from build123d import *

# Parameters (mm, degrees)
BOSS_EXTRUDE1_DEPTH = 5
SKETCH2_W           = 1.6
SKETCH2_H           = 1.6
CUT_EXTRUDE1_DEPTH  = 0.3
FILLET1_R           = 0.5


with BuildPart() as part:
    # Sketch1 → Boss-Extrude1 (new body)
    with BuildSketch(Plane(origin=(0, 0, 0), x_dir=(0, 0, -1), z_dir=(1, 0, 0))):
        with BuildLine():
            Line((-5.181029882, 3.015192247), (-4, 2.806944814))
            Line((-4, 2.806944814), (0.163235541, 2.072854061))
            ThreePointArc((0.163235541, 2.072854061), (0.459433673, 1.901843989), (0.576411452, 1.580450184))
            Line((0.576411452, 1.580450184), (0.576411452, 1.5))
            ThreePointArc((0.576411452, 1.5), (0.429964842, 1.146446609), (0.076411452, 1))
            Line((0.076411452, 1), (-6.25, 1))
            Line((-6.25, 1), (-6.25, 0))
            Line((-6.25, 0), (-4.8, 0))
            Line((-4.8, 0), (-4.8, -0.3))
            Line((-4.8, -0.3), (-3.2, -0.3))
            Line((-3.2, -0.3), (-3.2, 0))
            Line((-3.2, 0), (-1, 0))
            Line((-1, 0), (-1, -0.5))
            Line((-1, -0.5), (0, -0.5))
            Line((0, -0.5), (0, 0))
            ThreePointArc((0, 0), (1.536997065, 1.222015685), (0.692851848, 2.994895028))
            Line((0.692851848, 2.994895028), (-5.007381704, 4))
            Line((-5.007381704, 4), (-5.181029882, 3.015192247))
        make_face()
    extrude(amount=BOSS_EXTRUDE1_DEPTH)

    # Sketch2 → Cut-Extrude1 (cut)
    with BuildSketch(Plane.XZ.offset(0.3)):
        with Locations((2.5, 4)):
            Rectangle(SKETCH2_W, SKETCH2_H)
    extrude(amount=-CUT_EXTRUDE1_DEPTH, mode=Mode.SUBTRACT)

    # Fillet1
    fillet1_edges = [part.edges().sort_by_distance(p)[0] for p in [
        (0, 0.5, 6.25),
        (0, 3.507596123, 5.094205793),
        (5, 3.507596123, 5.094205793),
        (5, 0.5, 6.25),
    ]]
    fillet(fillet1_edges, radius=FILLET1_R)


solid = part.part
Part model, mm, in its own coordinate system. A direction names the side the tool comes from. Round coordinates to 2 decimals unless told otherwise and drop trailing zeros. Write each loop counter-clockwise with the first axis right and the second up, starting at its lowest first coordinate (ties: lowest second). Pieces come first, ordered by that corner, then holes. Notation, with made-up numbers: (48, 44.25) - (72, 44.25) arc R17 cw to (72, 48.25) - close; hole circle Ø3 at (38.5, 88). An arc over 180 degrees is marked (long way). Use CSV: the item, a comma, the result in double quotes.
Item 1: Slice it at A-A, the plane x = 3.05. Write the cut outline in (y, z), then the cut area to 3 significant figures.
Results list:
outline,"(-0.5, 0) - (0, 0) arc R1.58 ccw to (2.99, -0.69) - (4, 5.01) - (3.02, 5.18) - (2.07, -0.16) arc R0.5 cw to (1.58, -0.58) - (1.5, -0.58) arc R0.5 cw to (1, -0.08) - (1, 6.25) - (0, 6.25) - (0, 1) - (-0.5, 1) - close"
area,"15.3 mm²"
Item 2: Flat gauge pins, fed straight in: P1, Ø1, axis at x = 2, z = 0, coming from the +Y side; P2, Ø2.5, axis at x = 1.5, z = 3.5, coming from the -Y side; P3, Ø1, axis at x = 2, y = 2, coming from the -Z side; P4, Ø0.6, axis at x = 3.5, y = 0, coming from the -Z side. Where does each tip first touch, or does it go through?
Results list:
P1,"stops at y = 3.21"
P2,"stops at y = -0.3"
P3,"stops at z = -1.58"
P4,"stops at z = -0.93"
Item 3: Slice it at C-C, the plane x = 3.6. Write the cut outline in (y, z).
Results list:
outline,"(-0.5, 0) - (0, 0) arc R1.58 ccw to (2.99, -0.69) - (4, 5.01) - (3.02, 5.18) - (2.07, -0.16) arc R0.5 cw to (1.58, -0.58) - (1.5, -0.58) arc R0.5 cw to (1, -0.08) - (1, 6.25) - (0, 6.25) - (0, 4.8) - (-0.3, 4.8) - (-0.3, 3.2) - (0, 3.2) - (0, 1) - (-0.5, 1) - close"
Item 4: Slice it at D-D, the plane y = 0.4. Write the cut outline in (x, z).
Results list:
outline,"(0, -1.05) - (5, -1.05) - (5, 5.75) arc R0.5 ccw to (4.5, 6.25) - (0.5, 6.25) arc R0.5 ccw to (0, 5.75) - close"
Item 5: Pull direction Y, two halves, no side cores. Call faces 1 (the flat face through (2.472, 3.514, 5.093)), 2 (the flat face through (4, -0.3, 4)), 3 (the flat face through (2, 1, 3)): pulls with the +Y half, pulls with the -Y half, needs draft (parallel to the pull), parting line crosses it, or undercut.
Results list:
face 1,"pulls with the +Y half"
face 2,"pulls with the -Y half"
face 3,"undercut"
Item 6: Slice it at B-B, the plane z = 2. Write the cut outline in (x, y).
Results list:
outline,"(0, 0) - (5, 0) - (5, 1) - (0, 1) - close; (0, 2.45) - (5, 2.45) - (5, 3.47) - (0, 3.47) - close"
Item 7: Wall check: L1, parallel to Y at x = 3.25, z = 4; L2, parallel to Y at x = 3.05, z = 4.75; L3, parallel to Y at x = 3.1, z = 5.75. Give the ranges that are in metal, low to high.
Results list:
L1,"y = 0 to 1, 2.81 to 3.82"
L2,"y = 0 to 1, 2.94 to 3.95"
L3,"y = 0 to 1"
Item 8: Tool access for faces 4 (the flat face through (2.5, 0.5, 6.25)), 5 (the flat face through (1, -0.3, 4)): list every direction of +Z, -Z, +X, -X, +Y, -Y with a clear straight run to the whole face (end or side of a thin tool).
Results list:
face 4,"+Z, +X, -X, +Y, -Y"
face 5,"+Z, +X, -X, -Y"
